from build123d import *

# Parameters (mm, degrees)
BOSS_EXTRUDE1_DEPTH             = 3.175
SKETCH2_W                       = 2.75
SKETCH2_H                       = 2.5
SKETCH2_H_2                     = 4
SKETCH2_W_2                     = 1.125
SKETCH2_H_3                     = 7.5
CUT_EXTRUDE1_DEPTH              = 204.460831631
CIRPATTERN1_COUNT               = 2
CIRPATTERN1_ANGLE               = 65
CIRPATTERN1_THE_OTHER_WAY_COUNT = 2
CIRPATTERN1_THE_OTHER_WAY_ANGLE = 65
F_3_0_3_DIAMETER_HOLE1_D        = 3
F_8_0_8_DIAMETER_HOLE1_D        = 8
F_8_0_8_DIAMETER_HOLE1_DEPTH    = 6.35
F_8_CLEARANCE_HOLE1_D           = 4.4958
F_8_CLEARANCE_HOLE1_DEPTH       = 12.83
F_8_CLEARANCE_HOLE1_TIP         = 1.350674586
F_3_16_0_1875_DOWEL_HOLE1_D     = 4.7625
F_3_16_0_1875_DOWEL_HOLE1_DEPTH = 12.83
F_3_16_0_1875_DOWEL_HOLE1_TIP   = 1.430799349


with BuildPart() as part:
    # Sketch1 → Boss-Extrude1 (new, symmetric)
    with BuildSketch(Plane(origin=(0, 0, 0), x_dir=(1, 0, 0), z_dir=(0, 1, 0))):
        with BuildLine():
            Line((79.85, 28.959332111), (138.254290129, 56.193699868))
            ThreePointArc((138.254290129, 56.193699868), (0, 149.238), (-138.254290129, 56.193699868))
            Line((-138.254290129, 56.193699868), (-53.95, 16.881963765))
            Line((-53.95, 16.881963765), (-53.95, -38.1))
            Line((-53.95, -38.1), (79.85, -38.1))
            Line((79.85, -38.1), (79.85, 28.959332111))
        make_face()
        with BuildLine():
            Line((-7.5, 11.821590418), (-7.5, 11.772641828))
            Line((-7.5, 11.772641828), (-7.544362488, 11.793328396))
            ThreePointArc((-7.544362488, 11.793328396), (-7.522194517, 11.807480241), (-7.5, 11.821590418))
        make_face(mode=Mode.SUBTRACT)
        with BuildLine():
            ThreePointArc((7.5, 11.821590418), (7.522194517, 11.807480241), (7.544362488, 11.793328396))
            Line((7.544362488, 11.793328396), (7.5, 11.772641828))
            Line((7.5, 11.772641828), (7.5, 11.821590418))
        make_face(mode=Mode.SUBTRACT)
        with BuildLine():
            Line((-7.5, 134.028320306), (-7.5, 38.1))
            Line((-7.5, 38.1), (-53.95, 38.1))
            Line((-53.95, 38.1), (-53.95, 33.43263255))
            Line((-53.95, 33.43263255), (-118.301273414, 63.440124154))
            ThreePointArc((-118.301273414, 63.440124154), (-72.126024825, 113.215180903), (-7.5, 134.028320306))
        make_face(mode=Mode.SUBTRACT)
        with BuildLine():
            ThreePointArc((7.5, 134.028320306), (72.126024825, 113.215180903), (118.301273414, 63.440124154))
            Line((118.301273414, 63.440124154), (63.959201798, 38.1))
            Line((63.959201798, 38.1), (7.5, 38.1))
            Line((7.5, 38.1), (7.5, 134.028320306))
        make_face(mode=Mode.SUBTRACT)
    extrude(amount=BOSS_EXTRUDE1_DEPTH, both=True)

    # Sketch2 → Cut-Extrude1 (cut, symmetric)
    with BuildSketch(Plane(origin=(0, 0, 0), x_dir=(1, 0, 0), z_dir=(0, 1, 0))):
        with Locations((0, 136.488)):
            Rectangle(SKETCH2_W, SKETCH2_H)
        with Locations((0, 139.738)):
            Rectangle(SKETCH2_W, SKETCH2_H_2)
        with Locations((1.9375, 139.738)):
            Rectangle(SKETCH2_W_2, SKETCH2_H_2)
        with Locations((0, 145.488)):
            Rectangle(SKETCH2_W, SKETCH2_H_3)
        with Locations((-1.9375, 139.738)):
            Rectangle(SKETCH2_W_2, SKETCH2_H_2)
    cut_extrude1 = extrude(amount=CUT_EXTRUDE1_DEPTH, both=True, mode=Mode.SUBTRACT)

    # CirPattern1: Cut-Extrude1 ×2 about axis
    cirpattern1_axis = Axis((0, 0, 0), (0, 1, 0))
    for i in range(1, CIRPATTERN1_COUNT):
        add(cut_extrude1.rotate(cirpattern1_axis, i * CIRPATTERN1_ANGLE / (CIRPATTERN1_COUNT - 1)), mode=Mode.SUBTRACT)

    # CirPattern1 the other way: Cut-Extrude1 ×2 about axis
    cirpattern1_the_other_way_axis = Axis((0, 0, 0), (0, -1, 0))
    for i in range(1, CIRPATTERN1_THE_OTHER_WAY_COUNT):
        add(cut_extrude1.rotate(cirpattern1_the_other_way_axis, i * CIRPATTERN1_THE_OTHER_WAY_ANGLE / (CIRPATTERN1_THE_OTHER_WAY_COUNT - 1)), mode=Mode.SUBTRACT)

    # Ø3.0 (3) Diameter Hole1 (through all)
    with Locations(Plane(origin=(0, 3.175, 0), x_dir=(1, 0, 0), z_dir=(0, 1, 0))):
        with Locations((0, 0), (-76.155771888, 119.540616747), (76.155771888, 119.540616747), (69.85, 28.1), (69.85, -28.1), (-43.95, -28.1), (-43.95, 28.1)):
            Hole(F_3_0_3_DIAMETER_HOLE1_D / 2)

    # Ø8.0 (8) Diameter Hole1
    with Locations(Plane(origin=(0, 3.175, 0), x_dir=(1, 0, 0), z_dir=(0, 1, 0))):
        with Locations((0, 0)):
            Hole(F_8_0_8_DIAMETER_HOLE1_D / 2, depth=F_8_0_8_DIAMETER_HOLE1_DEPTH)

    # #8 Clearance Hole1
    with Locations(Plane(origin=(0, 3.175, 0), x_dir=(1, 0, 0), z_dir=(0, 1, 0))):
        with Locations((-50.775, -20), (-50.775, 20), (76.675, -20), (76.675, 20)):
            Hole(F_8_CLEARANCE_HOLE1_D / 2, depth=F_8_CLEARANCE_HOLE1_DEPTH)
            with Locations((0, 0, -(F_8_CLEARANCE_HOLE1_DEPTH + F_8_CLEARANCE_HOLE1_TIP / 2))):  # 118° drill point
                Cone(0, F_8_CLEARANCE_HOLE1_D / 2, F_8_CLEARANCE_HOLE1_TIP, mode=Mode.SUBTRACT)

    # 3/16 (0.1875) Dowel Hole1
    with Locations(Plane(origin=(0, 3.175, 0), x_dir=(1, 0, 0), z_dir=(0, 1, 0))):
        with Locations((-50.775, -10), (-50.775, 10), (76.675, -10), (76.675, 10)):
            Hole(F_3_16_0_1875_DOWEL_HOLE1_D / 2, depth=F_3_16_0_1875_DOWEL_HOLE1_DEPTH)
            with Locations((0, 0, -(F_3_16_0_1875_DOWEL_HOLE1_DEPTH + F_3_16_0_1875_DOWEL_HOLE1_TIP / 2))):  # 118° drill point
                Cone(0, F_3_16_0_1875_DOWEL_HOLE1_D / 2, F_3_16_0_1875_DOWEL_HOLE1_TIP, mode=Mode.SUBTRACT)


solid = part.part
Design review of the part built by this model. Coordinates are the model's own, in mm. A direction names the side the tool comes from. Coordinates: 2 decimals unless noted, no trailing zeros. Loops run counter-clockwise (first coordinate to the right, second up) from the corner with the lowest first, then second, coordinate; pieces in that order, holes last. Notation, with made-up numbers: (7, 23.5) -> (33, 23.5) arc R11 ccw to (33, 36.5) -> close; hole circle Ø4 at (4.25, 17). An arc over 180 degrees is marked (long way). Use a Markdown table: item, result. Add a question column.
Item 1: Machinability: for faces 1 (the flat face through (1.375, 0, -145)), 2 (the cylindrical face through (71.31, 0.04, -113.73)), 3 (the flat face through (108.643, 0.044, -42.386)), which of the approach directions +Z, -Z, +X, -X, +Y, -Y give a long, thin tool a straight path to every point of the face, cutting with its end or side? Answer none if there is none.
Item 2: The part is to be moulded in two halves that separate along X. For faces 4 (the cylindrical face through (-79.2, 0.04, -126.49)), 5 (the flat face through (-1.375, 0, -146)), 6 (the flat face through (79.85, 0, 5)), say which applies: +X half, -X half, draft (parallel to the pull), parting line (faces both ways), or undercut.
Item 3: We need section A-A, the plane x = 110. Write out the cut boundary in (y, z) (1 decimal), and give its area (3 significant figures).
Item 4: We need section C-C, the plane z = -126. Write out the cut boundary in (x, y) (3 decimals).
Item 5: Wall thickness on L1, parallel to X at y = -1.25, z = 10; L2, parallel to X at y = 0.25, z = 20; L3, parallel to Z at x = -52.5, y = -1: over which ranges is each line inside the solid? List them lowest first. Write a range as from..to.
Item 6: We need section B-B, the plane z = 0. Write out the cut boundary in (x, y) (3 decimals).
Item 7: Clearance check with flat-ended pins moving along their axes: P1, Ø2, axis at x = -46, y = 0, coming from the -Z side; P2, Ø3, axis at y = 1, z = -68, coming from the -X side; P3, Ø3, axis at x = 76.675, z = 10, coming from the +Y side; P4, Ø2, axis at y = 0, z = -136, coming from the +X side. State where each tip first meets the part, or that it passes through.
Numbers:
| question | item | result |
|---|---|---|
| 1 | face 1 | -Z, +Y, -Y |
| 1 | face 2 | +Y, -Y |
| 1 | face 3 | +Z, +X, +Y, -Y |
| 2 | face 4 | -X half |
| 2 | face 5 | undercut |
| 2 | face 6 | +X half |
| 3 | outline | (-3.2, -100.9) -> (3.2, -100.9) -> (3.2, -76.9) -> (-3.2, -76.9) -> close; (-3.2, -59.6) -> (3.2, -59.6) -> (3.2, -43) -> (-3.2, -43) -> close |
| 3 | area | 257 mm^2 |
| 4 | outline | (-79.975, -3.175) -> (-46.302, -3.175) -> (-46.302, 3.175) -> (-79.975, 3.175) -> close; (-7.5, -3.175) -> (7.5, -3.175) -> (7.5, 3.175) -> (-7.5, 3.175) -> close; (46.302, -3.175) -> (79.975, -3.175) -> (79.975, 3.175) -> (46.302, 3.175) -> close |
| 5 | L1 | x = -53.95..-53.16, -48.39..74.29, 79.06..79.85 |
| 5 | L2 | x = -53.95..-53.02, -48.53..74.43, 78.92..79.85 |
| 5 | L3 | z = -139.7..-123.55, -38.1..-21.44, -18.56..-11.64, -8.36..8.36, 11.64..18.56, 21.44..38.1 |
| 6 | outline | (-53.95, -3.175) -> (-4, -3.175) -> (-4, 3.175) -> (-53.95, 3.175) -> close; (4, -3.175) -> (79.85, -3.175) -> (79.85, 3.175) -> (4, 3.175) -> close |
| 7 | P1 | stops at z = -142.29 |
| 7 | P2 | stops at x = -133.6 |
| 7 | P3 | passes through |
| 7 | P4 | stops at x = 63.62 |
